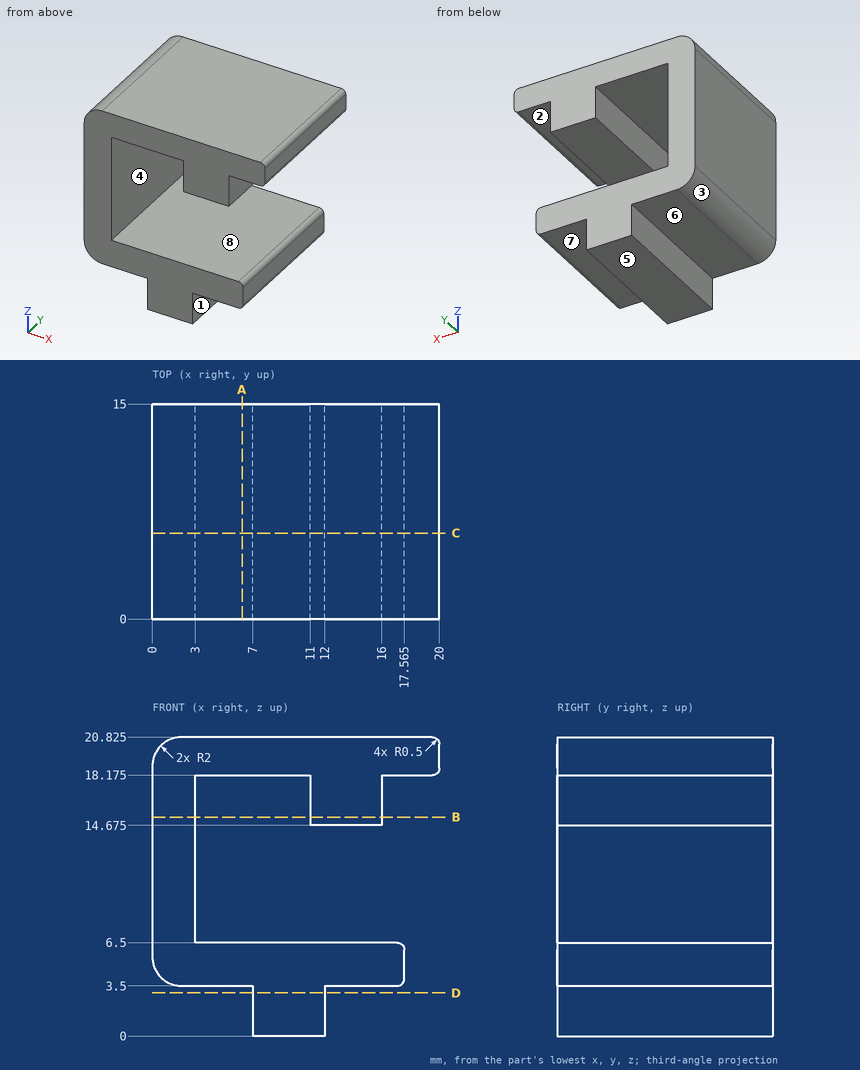
Drawing for the job (mm, zero at the part's lowest x, y, z). A direction names the side the tool comes from. Round coordinates to 2 decimals unless told otherwise and drop trailing zeros. Loops run counter-clockwise (first coordinate to the right, second up) from the corner with the lowest first, then second, coordinate; pieces in that order, holes last. Notation, with made-up numbers: M 56.5,46.5 L 76.5,46.5 A21 ccw 76.5,81.5 Z; hole C -11.75,30.25 d5. An arc over 180 degrees is marked long. Use a Markdown table: item, result. Add a question column.
(1) Drill centre lines: line 1 (Z direction, x = 8.75, y = 5.5) (1 decimal); line 2 (Z direction, x = 6.5, y = 3.75) (1 decimal); line 3 (X direction, y = 5.75, z = 18). Where is each one in solid material? Low to high.
(2) Which spindle directions (+Z, -Z, +X, -X, +Y, -Y) get a long thin tool onto all of the face, cutting with end or side? Do the marked faces 4, 5, 6, 7 and 8. Say none if no direction does.
(3) Cut at C-C (y = 6). Give the cut face in (x, z) (1 decimal), and give its area (3 significant figures).
(4) Cut at A-A (x = 6.25). Give the cut face in (y, z) (1 decimal).
(5) Cut at B-B (z = 15.25). Give the cut face in (x, y).
(6) Flat gauge pins, fed straight in: pin 1 (1.8 mm diameter, centred on y = 6.5, z = 1, fed in from -X); pin 2 (2.5 mm diameter, centred on x = 13.5, y = 6.5, fed in from -Z); pin 3 (1 mm diameter, centred on y = 5, z = 16.5, fed in from +X). Where does each tip first touch, or does it go through?
(7) Pull direction Z, two halves, no side cores. Call the marked faces 1, 2 and 3: +Z half, -Z half, draft (parallel to the pull), parting line (faces both ways), or undercut.
(8) Cut at D-D (z = 3). Give the cut face in (x, y).
Geometry says:
| question | item | result |
|---|---|---|
| 1 | line 1 | z = 0 to 6.5, 18.2 to 20.8 |
| 1 | line 2 | z = 3.5 to 6.5, 18.2 to 20.8 |
| 1 | line 3 | x = 0 to 3, 11 to 16 |
| 2 | face 4 | +Y, -Y |
| 2 | face 5 | -Z, +X, -X, +Y, -Y |
| 2 | face 6 | -Z, -X, +Y, -Y |
| 2 | face 7 | -Z, +X, +Y, -Y |
| 2 | face 8 | +X, +Y, -Y |
| 3 | outline | M 0,5.5 A2 ccw 2,3.5 L 7,3.5 L 7,0 L 12,0 L 12,3.5 L 17.1,3.5 A0.5 ccw 17.6,4 L 17.6,6 A0.5 ccw 17.1,6.5 L 3,6.5 L 3,18.2 L 11,18.2 L 11,14.7 L 16,14.7 L 16,18.2 L 19.5,18.2 A0.5 ccw 20,18.7 L 20,20.3 A0.5 ccw 19.5,20.8 L 2,20.8 A2 ccw 0,18.8 Z |
| 3 | area | 174 mm² |
| 4 | outline | M 0,3.5 L 15,3.5 L 15,6.5 L 0,6.5 Z; M 0,18.2 L 15,18.2 L 15,20.8 L 0,20.8 Z |
| 5 | outline | M 0,0 L 3,0 L 3,15 L 0,15 Z; M 11,0 L 16,0 L 16,15 L 11,15 Z |
| 6 | pin 1 | stops at x = 7 |
| 6 | pin 2 | stops at z = 3.5 |
| 6 | pin 3 | stops at x = 16 |
| 7 | face 1 | draft |
| 7 | face 2 | undercut |
| 7 | face 3 | -Z half |
| 8 | outline | M 7,0 L 12,0 L 12,15 L 7,15 Z |
